The listing builds one solid part. Answer for the finished solid, in the listing's coordinates (mm). A direction names the side the tool comes from. Give positions to 0.01 mm unless a question says otherwise; leave off trailing zeros. Loops run counter-clockwise (first coordinate to the right, second up) from the corner with the lowest first, then second, coordinate; pieces in that order, holes last. Notation, with made-up numbers: M 37,53.5 L 82,53.5 A21 ccw 82,85.5 Z; hole C 12,4.5 d1. An arc over 180 degrees is marked long. One line per item, written item: value. Start each with the question number.
Q1. A cutting plane is placed at A-A, the plane z = 19.5. Determine the outline of the cut face in (x, y).
Q2. A cutting plane is placed at B-B, the plane z = 32. Determine the outline of the cut face in (x, y), and give its area (3 significant figures).
Q3. Flat-ended cylindrical pins translate along their axes: pin 1 (5 mm diameter, centred on x = -37.5, z = 45, fed in from -Y); pin 2 (12 mm diameter, centred on y = 23.5, z = 8, fed in from -X); pin 3 (1 mm diameter, centred on x = 7, y = 17, fed in from +Z); pin 4 (3 mm diameter, centred on x = 34.5, z = 8.5, fed in from -Y). Find the tip coordinate at first contact, or state that the pin passes through.
Q4. The mould has two halves that part along Z. Classify faces 3 (the flat face through (10.09, -39.34, 30.066)), 4 (the flat face through (0, -45, 50.8)), 5 (the flat face through (0, 0, 0)): +Z half, -Z half, draft (parallel to the pull), parting line (faces both ways), or undercut.
Q5. For faces 1 (the conical face through (32.844, 10.343, 17.739)), 2 (the flat face through (7.73, -30.13, 11.061)), determine the directions among +Z, -Z, +X, -X, +Y, -Y from which every point of the face is accessible in a straight line to the end or side of a thin tool.
Q6. Consider L1, parallel to Z at x = -4, y = 17.5; L2, parallel to X at y = 18, z = 29; L3, parallel to X at y = -33, z = 44. Determine where each line is inside the solid, lowest interval first.
from build123d import *


with BuildPart() as f1:
    # F0 (on Front) → F1 (revolve)
    with BuildSketch(Plane.XZ):
        Polygon((0, 5.334), (0, 0), (25.4, 0), (30.930716, 11.061433), (32.660495, 14.520989), (34.351828, 17.903656), (36.378811, 21.957622), (38.40592, 26.01184), (40.433155, 30.066309), (42.665875, 34.53175), (44.859473, 38.918946), (50.8, 50.8), (44.836407, 50.8), (22.103407, 5.334), align=None)
        Polygon((32.660495, 14.520989), (30.930716, 11.061433), (34.072268, 11.061433), align=None)
        Polygon((34.351828, 17.903656), (32.660495, 14.520989), (36.043372, 14.520989), align=None)
        Polygon((36.378811, 21.957622), (34.351828, 17.903656), (38.406046, 17.903656), align=None)
        Polygon((46.310384, 34.53175), (44.859473, 38.918946), (42.665875, 34.53175), align=None)
        Polygon((38.40592, 26.01184), (36.378811, 21.957622), (40.433281, 21.957622), align=None)
        Polygon((44.488129, 30.066309), (42.665875, 34.53175), (40.433155, 30.066309), align=None)
        Polygon((40.433155, 30.066309), (38.40592, 26.01184), (42.460642, 26.01184), align=None)
    revolve(axis=Axis((0, 0, 25.4), (0, 0, 1)))


solid = f1.part
Answer block:
1. outline: C 0,0 d75.22; hole C 0,0 d58.37
2. outline: C 0,0 d87.4; hole C 0,0 d70.87
2. area: 2,050 mm^2
3. pin 1: y = -33.27
3. pin 2: x = -28.72
3. pin 3: z = 5.33
3. pin 4: through
4. face 3: undercut
4. face 4: +Z half
4. face 5: -Z half
5. face 1: none
5. face 2: -Z
6. L1: 0 to 5.33
6. L2: -36.8 to -28.77, 28.77 to 36.8
6. L3: -34.03 to -25.06, 25.06 to 34.03
